```python
from build123d import *

# Parameters (mm, degrees)
SFAZOWANIE1_SIZE = 0.5


with BuildPart() as part:
    # Szkic1 → Obrót1 (revolve)
    with BuildSketch(Plane.XY):
        Polygon((0, 0), (0, 10), (5, 10), (5, 7), (62, 7), (62, 0), align=None)
    revolve(axis=Axis((62, 0, 0), (-1, 0, 0)))

    # Sfazowanie1
    sfazowanie1_edges = [part.edges().sort_by_distance(p)[0] for p in [
        (62, -7, 0),
        (5, -10, 0),
        (0, -10, 0),
    ]]
    chamfer(sfazowanie1_edges, length=SFAZOWANIE1_SIZE)


solid = part.part
```
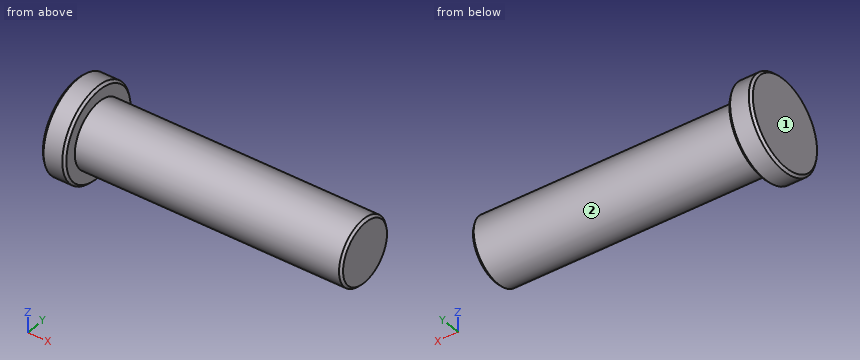
CAD build for the part. Positions are in the model's coordinates, mm. Face numbers are marked on the shaded views. A direction names the side the tool comes from. Coordinates: 2 decimals unless noted, no trailing zeros. Order: outer loops, then holes, each group sorted by start corner. A loop starts at its lowest first (then second) coordinate and runs counter-clockwise, first axis right, second up. Notation, with made-up numbers: M -1.5,75.5 L 56.5,75.5 A15 ccw 56.5,87.5 Z; hole C 79,71 d9. An arc over 180 degrees is marked long. Answer as CSV lines item,"result".
1) 3-axis set-ups, long thin cutter, end or side, ignore diameter. For the marked faces 1 and 2: which of +Z, -Z, +X, -X, +Y, -Y reach the whole face in a straight line?
Verdict:
face 1,"+Z, -Z, -X, +Y, -Y"
face 2,"+X"
2) Cut at C-C (x = 15). List the corners of the cut face in (y, z), then the cut area to 3 significant figures.
Verdict:
outline,"C 0,0 d14"
area,"154 mm2"
3) Cut at A-A (z = 0). List the corners of the cut face in (x, y).
Verdict:
outline,"M 0,-9.5 L 0.5,-10 L 4.5,-10 L 5,-9.5 L 5,-7 L 61.5,-7 L 62,-6.5 L 62,6.5 L 61.5,7 L 5,7 L 5,9.5 L 4.5,10 L 0.5,10 L 0,9.5 Z"
4) Drill centre lines: L1, parallel to Y at x = 8, z = 0; L2, parallel to X at y = -6.75, z = 4.5; L3, parallel to Y at x = 3.5, z = -0.5. Where is each one in solid material? Low to high. Write a range as from..to.
Verdict:
L1,"-7..7"
L2,"0..5"
L3,"-9.99..9.99"
5) Flat gauge pins, fed straight in: P1, Ø6, axis at y = 3.5, z = -7.5, coming from the -X side; P2, Ø5, axis at x = 23, z = -5, coming from the +Y side; P3, Ø1.5, axis at x = 27, y = 6, coming from the +Z side; P4, Ø1, axis at x = 21, y = -0.5, coming from the +Z side. Where does each tip first touch, or does it go through?
Verdict:
P1,"x = 0"
P2,"y = 6.54"
P3,"z = 4.63"
P4,"z = 7"
